Geometry: see drawing. Coordinates: mm, zero at the bounding-box minimum. Give positions to 0.01 mm unless a question says otherwise; leave off trailing zeros. Write each loop counter-clockwise with the first axis right and the second up, starting at its lowest first coordinate (ties: lowest second). Pieces come first, ordered by that corner, then holes. Notation, with made-up numbers: (-16, 48.25) -> (-5, 48.25) arc R24 ccw to (-5, 75.25) -> close; hole circle Ø4 at (9.5, -5). An arc over 180 degrees is marked (long way). Write item = value, one per line.
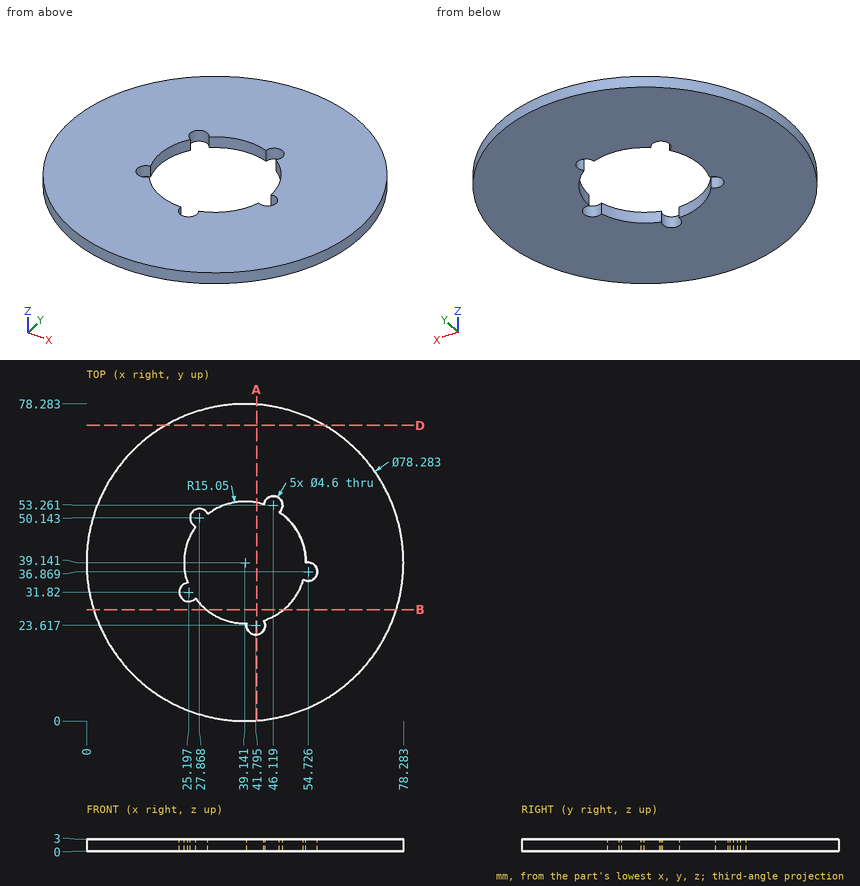
(1) Section query D-D (y = 73). Return loops of the section in (x, z), plus the area to 3 significant figures.
Values follow:
outline = (19.5, 0) -> (58.78, 0) -> (58.78, 3) -> (19.5, 3) -> close
area = 118 mm2
(2) Material intervals for line 1 (Y direction, x = 26.5, z = 0.2) (1 decimal); line 2 (Y direction, x = 54.5, z = 1.85) (1 decimal); line 3 (Y direction, x = 35, z = 1.75), sorted ascending.
Values follow:
line_1 = 2.1 to 29.9, 47.3 to 48.3, 52 to 76.2
line_2 = 3.1 to 34.6, 39.2 to 75.1
line_3 = 0.22 to 24.67, 53.61 to 78.06
(3) Section query B-B (y = 27.5). Return loops of the section in (x, z).
Values follow:
outline = (1.77, 0) -> (29.6, 0) -> (29.6, 3) -> (1.77, 3) -> close; (48.68, 0) -> (76.51, 0) -> (76.51, 3) -> (48.68, 3) -> close
(4) First-contact query: pin 1 (1 mm diameter, centred on x = 22, z = 1.5, fed in from +Y). Flat tip, straight axial feed; report the tip coordinate or a pass-through.
Values follow:
pin_1 = 74.57
(5) Section query A-A (x = 42). Return loops of the section in (y, z) (1 decimal).
Values follow:
outline = (0.1, 0) -> (21.3, 0) -> (21.3, 3) -> (0.1, 3) -> close; (53.9, 0) -> (78.2, 0) -> (78.2, 3) -> (53.9, 3) -> close
